Could you check a few things on this drawing? It's one solid part, dimensions in mm from its lowest x, y, z. A direction names the side the tool comes from. Give positions to 0.01 mm unless a question says otherwise; leave off trailing zeros. Order: outer loops, then holes, each group sorted by start corner. A loop starts at its lowest first (then second) coordinate and runs counter-clockwise, first axis right, second up. Notation, with made-up numbers: M 84.25,18.5 L 102.25,18.5 A13 ccw 102.25,23.5 Z; hole C -9,-16 d2. An arc over 180 degrees is marked long. Return JSON: item names as keys, results as strings. Group by question number.
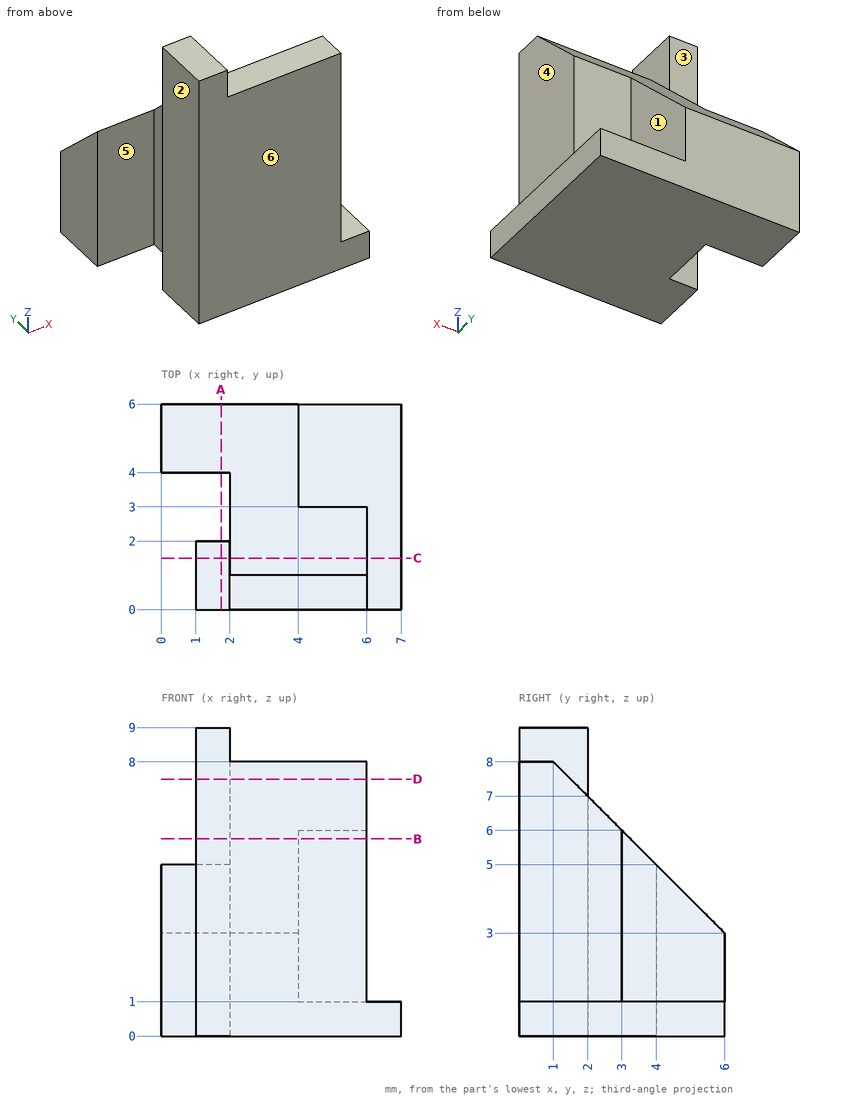
1. Imagine slicing it at A-A, the plane x = 1.75. Please give me the cut outline in (y, z).
2. Imagine slicing it at D-D, the plane z = 7.5. Please give me the cut outline in (x, y), plus the area to 3 significant figures.
3. Which directions (+Z, -Z, +X, -X, +Y, -Y) give clear straight access to the entire face, cutting with the end or side of a thin tool? Please do the marked faces 1, 2 and 3.
4. For pin 1 (0.5 mm diameter, centred on x = 1.5, z = 6.5, fed in from +Y); pin 2 (1.6 mm diameter, centred on x = 1, z = 3, fed in from -Y); pin 3 (1.5 mm diameter, centred on y = 2.5, z = 4, fed in from -X); pin 4 (3.5 mm diameter, centred on x = 6, y = 3.5, fed in from +Z), each with a flat end and sliding along its axis, tell me the tip position at first contact or that it passes through.
5. If we mould it in two halves opening along Y, with no side actions, what happens to the marked faces 4, 5 and 6? For each: pulls with the +Y half, pulls with the -Y half, needs draft (parallel to the pull), parting line crosses it, or undercut.
6. Imagine slicing it at B-B, the plane z = 5.75. Please give me the cut outline in (x, y).
7. Imagine slicing it at C-C, the plane y = 1.5. Please give me the cut outline in (x, z).
8. I need wall thicknesses on L1, parallel to Y at x = 1.5, z = 2.25; L2, parallel to Y at x = 5, z = 7; L3, parallel to X at y = 2.75, z = 2.5. Which ranges of each line are inside material? Lowest first, please. Write a range as from..to.
Values:
{
 "1": {"outline": "M 0,0 L 2,0 L 2,9 L 0,9 Z; M 4,0 L 6,0 L 6,3 L 4,5 Z"},
 "2": {"outline": "M 1,0 L 6,0 L 6,1.5 L 2,1.5 L 2,2 L 1,2 Z", "area": "8.00 mm²"},
 "3": {"face 1": "+Z, +X, +Y", "face 2": "+Z, -Z, -X, -Y", "face 3": "+Z, -Z, -X"},
 "4": {"pin 1": "stops at y = 2", "pin 2": "stops at y = 0", "pin 3": "stops at x = 1", "pin 4": "stops at z = 7.25"},
 "5": {"face 4": "needs draft", "face 5": "undercut", "face 6": "pulls with the -Y half"},
 "6": {"outline": "M 1,0 L 6,0 L 6,3 L 4,3 L 4,3.25 L 2,3.25 L 2,2 L 1,2 Z"},
 "7": {"outline": "M 1,0 L 7,0 L 7,1 L 6,1 L 6,7.5 L 2,7.5 L 2,9 L 1,9 Z"},
 "8": {"L1": "y = 0..2, 4..6", "L2": "y = 0..2", "L3": "x = 2..6"}
}
